from build123d import *

# Parameters (mm, degrees)
SKETCH1_W           = 40
SKETCH1_H           = 20
SKETCH1_R           = 3
BOSS_EXTRUDE1_DEPTH = 5
FILLET1_R           = 1


with BuildPart() as part:
    # Sketch1 → Boss-Extrude1 (new body)
    with BuildSketch(Plane(origin=(0, 0, 0), x_dir=(1, 0, 0), z_dir=(0, 1, 0))):
        Rectangle(SKETCH1_W, SKETCH1_H)
        with Locations((-15, 0)):
            Circle(SKETCH1_R, mode=Mode.SUBTRACT)
        with Locations((15, 0)):
            Circle(SKETCH1_R, mode=Mode.SUBTRACT)
        Circle(SKETCH1_R, mode=Mode.SUBTRACT)
    extrude(amount=BOSS_EXTRUDE1_DEPTH)

    # Fillet1
    fillet1_edges = [part.edges().sort_by_distance(p)[0] for p in [
        (20, 5, 0),
        (0, 5, -10),
        (-20, 5, 0),
        (0, 5, 10),
    ]]
    fillet(fillet1_edges, radius=FILLET1_R)


solid = part.part
CAD build for the part. Positions are in the model's coordinates, mm. Coordinates: 2 decimals unless noted, no trailing zeros. Loops run counter-clockwise (first coordinate to the right, second up) from the corner with the lowest first, then second, coordinate; pieces in that order, holes last. Notation, with made-up numbers: (51, 9) - (109, 9) arc R14 cw to (109, 23) - close; hole circle Ø7 at (80.25, 61.5). An arc over 180 degrees is marked (long way). Write item = value, one per line. Start each with the question number.
Q1. Flat gauge pins, fed straight in: pin 1 Ø8 at (x, z) = (-5.5, 4.5) entering from -Y; pin 2 Ø5 at (x, z) = (0, 0) entering from +Y. Where does each tip first touch, or does it go through?
Q2. Drill centre lines: L1, parallel to X at y = 3.55, z = 0; L2, parallel to Z at x = 0, y = 3.25; L3, parallel to X at y = 2.55, z = 2.5. Where is each one in solid material? Low to high.
Q3. Cut at C-C, the plane x = -15. List the corners of the cut face in (y, z), then the cut area to 3 significant figures.
Q4. Cut at B-B, the plane y = 1. List the corners of the cut face in (x, z).
Q5. Pull direction Z, two halves, no side cores. Call faces 1 (the flat face through (0, 2, -10)), 2 (the cylindrical face through (0.28, 4.699, 9.715)), 3 (the cylindrical face through (-18, 2, 0)), 4 (the flat face through (-5, 0, 0)): pulls with the +Z half, pulls with the -Z half, needs draft (parallel to the pull), parting line crosses it, or undercut.
Q6. Cut at A-A, the plane z = 0. List the corners of the cut face in (x, y), then the cut area to 3 significant figures.
Computed:
q1.pin_1 = 0
q1.pin_2 = through
q2.L1 = -20 to -18, -12 to -3, 3 to 12, 18 to 20
q2.L2 = -10 to -3, 3 to 10
q2.L3 = -20 to -16.66, -13.34 to -1.66, 1.66 to 13.34, 16.66 to 20
q3.outline = (0, -10) - (4, -10) arc R1 ccw to (5, -9) - (5, -3) - (0, -3) - close; (0, 3) - (5, 3) - (5, 9) arc R1 ccw to (4, 10) - (0, 10) - close
q3.area = 69.6 mm²
q4.outline = (-20, -10) - (20, -10) - (20, 10) - (-20, 10) - close; hole circle Ø6 at (-15, 0); hole circle Ø6 at (0, 0); hole circle Ø6 at (15, 0)
q5.face_1 = pulls with the -Z half
q5.face_2 = pulls with the +Z half
q5.face_3 = undercut
q5.face_4 = needs draft
q6.outline = (-20, 0) - (-18, 0) - (-18, 5) - (-19, 5) arc R1 ccw to (-20, 4) - close; (-12, 0) - (-3, 0) - (-3, 5) - (-12, 5) - close; (3, 0) - (12, 0) - (12, 5) - (3, 5) - close; (18, 0) - (20, 0) - (20, 4) arc R1 ccw to (19, 5) - (18, 5) - close
q6.area = 110 mm²
